```python
from build123d import *

# Parameters (mm, degrees)
F0_R = 48.75
F2_W = 68.9429111657
F2_H = 68.9429111657
F4_T = 2.5


# Not quite as in the source:
# - a shell that OpenCascade refuses in one call is made with other operations: the cavity is built on its own and cut out


with BuildPart() as f3:
    # F0 (on Top) → F3 section 0
    with BuildSketch(Plane.XY):
        Circle(F0_R)
    # F2 (on offset) → F3 section 1
    with BuildSketch(Plane.XY.offset(-30)):
        Rectangle(F2_W, F2_H)
    loft()

    # F4: shell of thickness 2.5, made by hand


with BuildPart() as f4_core1:
    # F4_t2: copy of F3
    add(f3.part)

    # the walls: a layer under each face that stays
    f4_faces = [f4_core1.faces().sort_by_distance(p)[0] for p in [
        (39.7552913915, 17.9457725576, -15),
        (0, 41.6107277896, -15),
        (-41.6107277896, 0, -15),
        (0, -41.6107277896, -15),
        (39.7552913915, -17.9457725576, -15),
        (0, 0, -30),
    ]]
    thicken(f4_faces, amount=-F4_T, mode=Mode.SUBTRACT)


with BuildPart() as f3_1:
    add(f3.part)

    # what is left inside the walls is the cavity
    f4_cavity = [f4_core1.part.solids().sort_by_distance(p)[0] for p in [
        (0, -15.327093, -0.025),
    ]]
    add(f4_cavity, mode=Mode.SUBTRACT)


solid = f3_1.part
```
CAD build for the part. Positions are in the model's coordinates, mm. Round coordinates to 2 decimals unless told otherwise and drop trailing zeros. One line per question, with ' | ' between items.
Q1. Two-plate mould, pull along Y, no slides. Class faces 1 (the flat face through (0, -1, -27.5)), 2 (the flat face through (0, -1, -30)): released by +Y, released by -Y, zero draft, split by the parting line, or undercut.
Completed:
face 1: undercut | face 2: zero draft
Q2. Drop flat-ended pins along their axis: pin 1 (10 mm diameter, centred on y = -5.5, z = -9.5, fed in from -X); pin 2 (4 mm diameter, centred on y = -18.5, z = -10, fed in from +X); pin 3 (1 mm diameter, centred on x = 17.5, z = -5, fed in from -Y). Give the stop position or say it passes through.
Completed:
pin 1: stops at x = -46.38 | pin 2: stops at x = 42.36 | pin 3: stops at y = -43.84
Q3. Probe probe 1 along Y at (x, z) = (-23, -9); probe 2 along Y at (x, z) = (-22.5, -16); probe 3 along Z at (x, y) = (30, -23.5). List the from-to ranges inside material, lowest first.
Completed:
probe 1: y = -40.27 to -37.5, 37.5 to 40.27 | probe 2: y = -38.38 to -35.71, 35.71 to 38.38 | probe 3: z = -30 to -27.5
